Design review of the part built by this model. Coordinates are the model's own, in mm. Give positions to 0.01 mm unless a question says otherwise; leave off trailing zeros. Order: outer loops, then holes, each group sorted by start corner. A loop starts at its lowest first (then second) coordinate and runs counter-clockwise, first axis right, second up. Notation, with made-up numbers: (18, -13) -> (23, -13) arc R16 cw to (23, 9) -> close; hole circle Ø10 at (-4.5, 24.25). An arc over 180 degrees is marked (long way). Return JSON: item names as keys, results as strings.
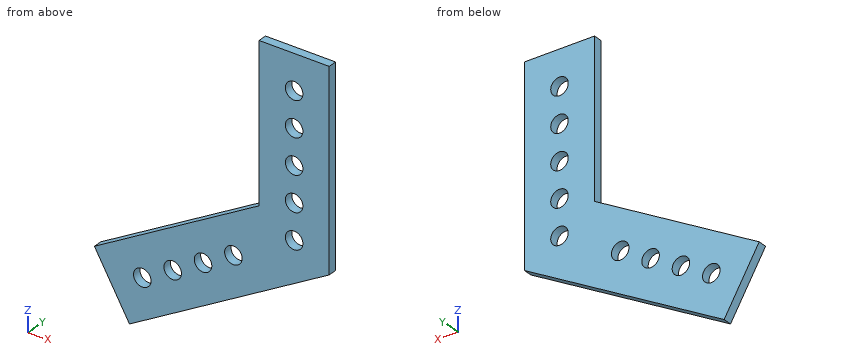
```python
from build123d import *

# Parameters (mm, degrees)
BOSS_EXTRUDE1_DEPTH = 3.175
SKETCH2_R           = 3.175
CUT_EXTRUDE1_DEPTH  = 97.30976352


with BuildPart() as part:
    # Sketch1 → Boss-Extrude1 (new body)
    with BuildSketch(Plane(origin=(0, 0, 0), x_dir=(1, 0, 0), z_dir=(0, 1, 0))):
        Polygon((12.7, 7.332348419), (12.7, -63.5), (-12.7, -63.5), (-12.7, -7.332348419), (-72.341135768, 27.101477372), (-59.641135768, 49.098522628), align=None)
    extrude(amount=BOSS_EXTRUDE1_DEPTH)

    # Sketch2 → Cut-Extrude1 (cut, through all)
    with BuildSketch(Plane(origin=(0, 3.175, 0), x_dir=(1, 0, 0), z_dir=(0, 1, 0))):
        with Locations(Location((-54.99261314, 31.75, 0), (0, 0, 270))):
            Circle(SKETCH2_R)
        with Locations(Location((-43.994090512, 25.4, 0), (0, 0, 270))):
            Circle(SKETCH2_R)
        with Locations(Location((-32.995567884, 19.05, 0), (0, 0, 270))):
            Circle(SKETCH2_R)
        with Locations(Location((-21.997045256, 12.7, 0), (0, 0, 270))):
            Circle(SKETCH2_R)
        with Locations(Location((0, 0, 0), (0, 0, 270))):
            Circle(SKETCH2_R)
        with Locations(Location((0, -50.8, 0), (0, 0, 270))):
            Circle(SKETCH2_R)
        with Locations(Location((0, -38.1, 0), (0, 0, 270))):
            Circle(SKETCH2_R)
        with Locations(Location((0, -25.4, 0), (0, 0, 270))):
            Circle(SKETCH2_R)
        with Locations(Location((0, -12.7, 0), (0, 0, 270))):
            Circle(SKETCH2_R)
    extrude(amount=-CUT_EXTRUDE1_DEPTH, mode=Mode.SUBTRACT)


solid = part.part
```
Item 1: Add section C-C (y = 2.2). Give the number of separate pieces and of enclosed holes in the cut face, plus the area to 3 significant figures.
Result set:
{"separate pieces": "1", "enclosed holes": "9", "area": "3,260 mm^2"}
Item 2: Add section A-A (z = 12.7). Give the boundary of the cut face in (x, y) (3 decimals), plus the area to 3 significant figures.
Result set:
{"outline": "(-12.7, 0) -> (-3.175, 0) -> (-3.175, 3.175) -> (-12.7, 3.175) -> close; (3.175, 0) -> (12.7, 0) -> (12.7, 3.175) -> (3.175, 3.175) -> close", "area": "60.5 mm^2"}
Item 3: Wall thickness on L1, parallel to X at y = 1.5, z = 25.4 (3 decimals); L2, parallel to Z at x = -35, y = 0.7; L3, parallel to X at y = 1.25, z = -2.5: over which ranges is each line inside the solid? List them lowest first. Write a range as [from, to].
Result set:
{"L1": "x = [-12.7, -3.175], [3.175, 12.7]", "L2": "z = [-34.87, -21.51], [-16.59, -5.54]", "L3": "x = [-29.73, -1.96], [1.96, 12.7]"}
Item 4: For pin 1 (1.5 mm diameter, centred on x = -42, y = 2, fed in from +Z); pin 2 (10 mm diameter, centred on x = -54.99, z = -31.75, fed in from -Y); pin 3 (1.6 mm diameter, centred on y = 1.5, z = 48.5, fed in from -X), all flat-tipped, find the tip position at first contact; note any pin that passes through.
Result set:
{"pin 1": "stops at z = -9.15", "pin 2": "stops at y = 0", "pin 3": "stops at x = -12.7"}
Item 5: Add section B-B (x = 0). Give the boundary of the cut face in (y, z) (3 decimals), plus the area to 3 significant figures.
Result set:
{"outline": "(0, -14.665) -> (3.175, -14.665) -> (3.175, -3.175) -> (0, -3.175) -> close; (0, 3.175) -> (3.175, 3.175) -> (3.175, 9.525) -> (0, 9.525) -> close; (0, 15.875) -> (3.175, 15.875) -> (3.175, 22.225) -> (0, 22.225) -> close; (0, 28.575) -> (3.175, 28.575) -> (3.175, 34.925) -> (0, 34.925) -> close; (0, 41.275) -> (3.175, 41.275) -> (3.175, 47.625) -> (0, 47.625) -> close; (0, 53.975) -> (3.175, 53.975) -> (3.175, 63.5) -> (0, 63.5) -> close", "area": "147 mm^2"}
Item 6: Add section D-D (z = -31.75). Give the boundary of the cut face in (x, y) (3 decimals).
Result set:
{"outline": "(-69.657, 0) -> (-58.168, 0) -> (-58.168, 3.175) -> (-69.657, 3.175) -> close; (-51.818, 0) -> (-29.593, 0) -> (-29.593, 3.175) -> (-51.818, 3.175) -> close"}
